```python
from build123d import *

# Parameters (mm, degrees)
BOSS_EXTRUDE1_DEPTH = 25.4
SKETCH2_R           = 3.3782
CUT_EXTRUDE1_DEPTH  = 25.4
SKETCH3_R           = 3.3782
CUT_EXTRUDE2_DEPTH  = 128.310769772
BOSS_EXTRUDE2_DEPTH = 25.4


with BuildPart() as part:
    # Sketch1 → Boss-Extrude1 (new body)
    with BuildSketch(Plane.XY):
        Polygon((0, 3.175), (0, 0), (3.175, 0), (101.6, 0), (101.6, 3.175), (3.175, 3.175), (3.175, 72.39), (0, 72.39), align=None)
    extrude(amount=BOSS_EXTRUDE1_DEPTH)

    # Sketch2 → Cut-Extrude1 (cut)
    with BuildSketch(Plane(origin=(0, 3.175, 0), x_dir=(1, 0, 0), z_dir=(0, 1, 0))):
        with Locations(Location((88.9, -12.7, 0), (0, 0, 270))):
            Circle(SKETCH2_R)
        with Locations(Location((25.4, -12.7, 0), (0, 0, 270))):
            Circle(SKETCH2_R)
    extrude(amount=-CUT_EXTRUDE1_DEPTH, mode=Mode.SUBTRACT)

    # Sketch3 → Cut-Extrude2 (cut, through all)
    with BuildSketch(Plane.ZY):
        with Locations((12.7, 27.94)):
            Circle(SKETCH3_R)
        with Locations((12.7, 46.99)):
            Circle(SKETCH3_R)
        with Locations((12.7, 66.04)):
            Circle(SKETCH3_R)
    extrude(amount=-CUT_EXTRUDE2_DEPTH, mode=Mode.SUBTRACT)

    # Sketch4 → Boss-Extrude2 (add)
    with BuildSketch(Plane.XY.offset(25.4)):
        Polygon((3.175, 14.605), (14.605, 3.175), (3.175, 3.175), align=None)
    extrude(amount=-BOSS_EXTRUDE2_DEPTH)


solid = part.part
```
Geometry check sheet. Reference: the model listing, model coordinates, mm. A direction names the side the tool comes from. Round coordinates to 2 decimals unless told otherwise and drop trailing zeros. Write each loop counter-clockwise with the first axis right and the second up, starting at its lowest first coordinate (ties: lowest second). Pieces come first, ordered by that corner, then holes. Notation, with made-up numbers: (15, -24) -> (54, -24) arc R25 ccw to (54, 4) -> close; hole circle Ø1 at (62, -25.75). An arc over 180 degrees is marked (long way). Put each result on its own line as item: value.
1) Cross-section at C-C, the plane z = 19.5. Enter the section's corners in (x, y) (3 decimals), plus the area to 3 significant figures.
Recorded:
outline: (0, 0) -> (101.6, 0) -> (101.6, 3.175) -> (14.605, 3.175) -> (3.175, 14.605) -> (3.175, 72.39) -> (0, 72.39) -> close
area: 608 mm2
2) Thickness scan on probe 1 along X at (y, z) = (2.2, 12.7); probe 2 along Y at (x, z) = (1.3, 12.7); probe 3 along X at (y, z) = (24.5, 11.5) (3 decimals). Record the ranges inside material, lowest first. Write a range as from..to.
Recorded:
probe 1: x = 0..22.02, 28.78..85.52, 92.28..101.6
probe 2: y = 0..24.56, 31.32..43.61, 50.37..62.66, 69.42..72.39
probe 3: x = 0..3.175
3) Cross-section at D-D, the plane y = 7. Enter the section's corners in (x, z).
Recorded:
outline: (0, 0) -> (10.78, 0) -> (10.78, 25.4) -> (0, 25.4) -> close
4) Release check for a two-part mould opening along Y. For faces 1 (the face through (92.25, 1.61, 12.26)), 2 (the face through (8.81, 8.97, 12.88)), 3 (the face through (1.57, 31.29, 12.26)), 4 (the face through (1.57, 43.69, 11.97)) record: pulls with the +Y half, pulls with the -Y half, needs draft (parallel to the pull), parting line crosses it, or undercut.
Recorded:
face 1: needs draft
face 2: pulls with the +Y half
face 3: undercut
face 4: undercut
5) Access from +Z, -Z, +X, -X, +Y, -Y to the whole of each face (thin tool, end or side, straight path). Record for faces 5 (the face through (59, 3.175, 13)), 6 (the face through (0, 37, 13)).
Recorded:
face 5: +Z, -Z, +X, +Y
face 6: +Z, -Z, -X, +Y, -Y
6) Depth check by flat-ended pin: P1, Ø9, axis at y = 27.94, z = 12.7, coming from the +X side (3 decimals); P2, Ø1, axis at y = 57, z = 5.5, coming from the -X side; P3, Ø6, axis at x = 71, z = 12.5, coming from the +Y side (3 decimals). Enter the tip coordinate at first touch or a pass-through.
Recorded:
P1: stops at x = 3.175
P2: stops at x = 0
P3: stops at y = 3.175
7) Cross-section at A-A, the plane x = 88.9. Enter the section's corners in (y, z) (3 decimals), plus the area to 3 significant figures.
Recorded:
outline: (0, 0) -> (3.175, 0) -> (3.175, 9.322) -> (0, 9.322) -> close; (0, 16.078) -> (3.175, 16.078) -> (3.175, 25.4) -> (0, 25.4) -> close
area: 59.2 mm2
